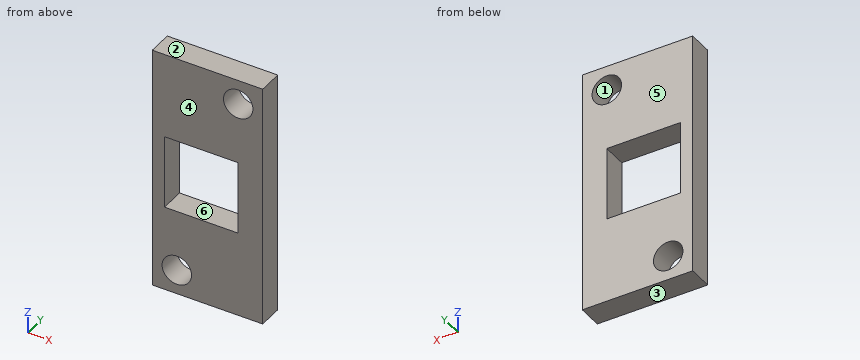
```python
from build123d import *

# Parameters (mm, degrees)
SKETCH_1_W              = 9
SKETCH_1_H              = 2
CARRIER_1_DEPTH         = 20
SKETCH_2_W              = 6
SKETCH_2_H              = 6
TACT_6X6_POCKET_2_DEPTH = 4
SKETCH_3_R              = 1.2
CARRIER_M2_3_DEPTH      = 4


with BuildPart() as part:
    # Эскиз1 → Carrier_1 (new body)
    with BuildSketch(Plane.XY.offset(67)):
        with Locations((38.5, -55)):
            Rectangle(SKETCH_1_W, SKETCH_1_H)
    extrude(amount=CARRIER_1_DEPTH)

    # Эскиз2 → Tact_6x6_pocket_2 (cut)
    with BuildSketch(Plane(origin=(0, -57, 0), x_dir=(1, 0, 0), z_dir=(0, 1, 0))):
        with Locations((38, -77)):
            Rectangle(SKETCH_2_W, SKETCH_2_H)
    extrude(amount=TACT_6X6_POCKET_2_DEPTH, mode=Mode.SUBTRACT)

    # Эскиз3 → Carrier_M2_3 (cut)
    with BuildSketch(Plane(origin=(0, -57, 0), x_dir=(1, 0, 0), z_dir=(0, 1, 0))):
        with Locations(Location((36, -69, 0), (0, 0, 90))):
            Circle(SKETCH_3_R)
        with Locations(Location((41, -85, 0), (0, 0, 90))):
            Circle(SKETCH_3_R)
    extrude(amount=CARRIER_M2_3_DEPTH, mode=Mode.SUBTRACT)


solid = part.part
```
Read the model definition and answer for the solid it produces. Units are mm, in the model's axes. Face numbers are marked on the shaded views. A direction names the side the tool comes from. Give positions to 0.01 mm unless a question says otherwise; leave off trailing zeros. Loops run counter-clockwise (first coordinate to the right, second up) from the corner with the lowest first, then second, coordinate; pieces in that order, holes last.
Item 1: The part is cut by section D-D (y = -54.3). Write down the section's boundary in (x, z).
Item 2: Find the intervals of material crossed by line 1 along X through (y, z) = (-54.8, 76.5); line 2 along Z through (x, y) = (38.5, -55.4); line 3 along X through (y, z) = (-54.8, 69), in increasing order.
Item 3: The part is cut by section B-B (x = 38.25). Write down the section's boundary in (y, z), and give its area (3 significant figures).
Item 4: The mould has two halves that part along Z. Classify the marked faces 1, 2, 3 and 4: released by +Z, released by -Z, zero draft, split by the parting line, or undercut.
Item 5: The part is cut by section A-A (x = 36). Write down the section's boundary in (y, z), and give its area (3 significant figures).
Item 6: The part is cut by section C-C (z = 69). Write down the section's boundary in (x, y).
Item 7: For the marked faces 5 and 6, determine the directions among +Z, -Z, +X, -X, +Y, -Y from which every point of the face is accessible in a straight line to the end or side of a thin tool.
Taken from the geometry:
1. outline: (34, 67) - (43, 67) - (43, 87) - (34, 87) - close; hole circle Ø2.4 at (36, 69); hole (35, 74) - (41, 74) - (41, 80) - (35, 80) - close; hole circle Ø2.4 at (41, 85)
2. line 1: x = 34 to 35, 41 to 43
2. line 2: z = 67 to 74, 80 to 87
2. line 3: x = 34 to 34.8, 37.2 to 43
3. outline: (-56, 67) - (-54, 67) - (-54, 74) - (-56, 74) - close; (-56, 80) - (-54, 80) - (-54, 87) - (-56, 87) - close
3. area: 28.0 mm2
4. face 1: undercut
4. face 2: released by +Z
4. face 3: released by -Z
4. face 4: zero draft
5. outline: (-56, 67) - (-54, 67) - (-54, 67.8) - (-56, 67.8) - close; (-56, 70.2) - (-54, 70.2) - (-54, 74) - (-56, 74) - close; (-56, 80) - (-54, 80) - (-54, 87) - (-56, 87) - close
5. area: 23.2 mm2
6. outline: (34, -56) - (34.8, -56) - (34.8, -54) - (34, -54) - close; (37.2, -56) - (43, -56) - (43, -54) - (37.2, -54) - close
7. face 5: +Z, -Z, +X, -X, +Y
7. face 6: +Y, -Y
